```python
from build123d import *

# Parameters (mm, degrees)
F0_R     = 19.05
F0_R_2   = 18.25625
F1_DEPTH = 50.8
F2_R     = 6.35
F3_DEPTH = 44.45
F0_R_3   = 6.35
F4_DEPTH = 38.1
F5_R     = 1.5875
F6_DEPTH = 31.75


with BuildPart() as f1:
    # F0 (on Front) → F1 (new body)
    with BuildSketch(Plane.XZ):
        Circle(F0_R)
        Circle(F0_R_2, mode=Mode.SUBTRACT)
    extrude(amount=F1_DEPTH)



with BuildPart() as f3:
    # F2 (on Front) → F3 (new body)
    with BuildSketch(Plane.XZ):
        Circle(F2_R)
    extrude(amount=F3_DEPTH)


with BuildPart() as f1_1:
    add(f1.part)

    add(f3.part)  # F4 merges F3
    # F0 (on Front) → F4 (join)
    with BuildSketch(Plane.XZ):
        Circle(F0_R_2)
        Circle(F0_R_3, mode=Mode.SUBTRACT)
    extrude(amount=F4_DEPTH)

    # F5 (on Front) → F6 (join)
    with BuildSketch(Plane.XZ):
        Circle(F5_R)
    extrude(amount=-F6_DEPTH)


solid = f1_1.part
```
Part model, mm, in its own coordinate system. A direction names the side the tool comes from. Coordinates: 2 decimals unless noted, no trailing zeros. Write each loop counter-clockwise with the first axis right and the second up, starting at its lowest first coordinate (ties: lowest second). Pieces come first, ordered by that corner, then holes.
Item 1: Slice it at B-B (z = 0). Write the cut outline in (x, y), and give its area (3 significant figures).
Item 2: Which spindle directions (+Z, -Z, +X, -X, +Y, -Y) get a long thin tool onto all of the face, cutting with end or side? Do faces 1 (the face through (-0.34, 15.65, -1.55)), 2 (the face through (0, -44.45, 0)). Say none if no direction does.
Item 3: Slice it at D-D (x = -16). Write the cut outline in (y, z).
Item 4: Slice it at C-C (y = 21). Write the cut outline in (x, z) (1 decimal).
Item 5: Mould opens along X. For faces 3 (the face through (0, 31.75, 0)), 4 (the face through (17.413, -44.361, 5.484)), 5 (the face through (-15.12, -25.04, -11.59)) say: released by +X, released by -X, zero draft, split by the parting line, or undercut.
Item 6: Slice it at A-A (x = 0). Write the cut outline in (y, z), and give its area (3 significant figures).
Item 7: Pin check, flat tips, straight feed: pin 1 (2 mm diameter, centred on x = 3, y = 1.5, fed in from -Z); pin 2 (8 mm diameter, centred on x = 14.5, y = -26, fed in from +Z); pin 3 (4 mm diameter, centred on y = 1.5, z = -8.5, fed in from -X); pin 4 (3 mm diameter, centred on y = -24.5, z = -3.5, fed in from -X). Stop position of each tip, or through.
Item 8: Probe line 1 (Z direction, x = 0, y = -42.5); line 2 (Z direction, x = 0, y = -47); line 3 (Y direction, x = 7, z = -14.5). List the from-to ranges inside material, lowest first.
Results found:
1. outline: (-19.05, -50.8) - (-18.26, -50.8) - (-18.26, -38.1) - (-6.35, -38.1) - (-6.35, -44.45) - (6.35, -44.45) - (6.35, -38.1) - (18.26, -38.1) - (18.26, -50.8) - (19.05, -50.8) - (19.05, 0) - (1.59, 0) - (1.59, 31.75) - (-1.59, 31.75) - (-1.59, 0) - (-19.05, 0) - close
1. area: 1,650 mm2
2. face 1: +Y
2. face 2: -Y
3. outline: (-50.8, -10.34) - (0, -10.34) - (0, 10.34) - (-50.8, 10.34) - (-50.8, 8.79) - (-38.1, 8.79) - (-38.1, -8.79) - (-50.8, -8.79) - close
4. outline: circle Ø3.2 at (0, 0)
5. face 3: zero draft
5. face 4: undercut
5. face 5: split by the parting line
6. outline: (-50.8, -19.05) - (0, -19.05) - (0, -1.59) - (31.75, -1.59) - (31.75, 1.59) - (0, 1.59) - (0, 19.05) - (-50.8, 19.05) - (-50.8, 18.26) - (-38.1, 18.26) - (-38.1, 6.35) - (-44.45, 6.35) - (-44.45, -6.35) - (-38.1, -6.35) - (-38.1, -18.26) - (-50.8, -18.26) - close
6. area: 1,650 mm2
7. pin 1: passes through
7. pin 2: stops at z = 15.9
7. pin 3: stops at x = -17.65
7. pin 4: stops at x = -18.94
8. line 1: z = -19.05 to -18.26, -6.35 to 6.35, 18.26 to 19.05
8. line 2: z = -19.05 to -18.26, 18.26 to 19.05
8. line 3: y = -38.1 to 0
